Here's how the part is built. I have some questions about the finished solid (model axes, mm). Face numbers are marked on the shaded views. Give positions to 0.01 mm unless a question says otherwise; leave off trailing zeros. Write each loop counter-clockwise with the first axis right and the second up, starting at its lowest first coordinate (ties: lowest second). Pieces come first, ordered by that corner, then holes. Notation, with made-up numbers: (51, 27) - (97, 27) arc R33 ccw to (97, 60) - close; hole circle Ø3 at (77.5, -33.75). An arc over 180 degrees is marked (long way). Use a Markdown table: item, result.
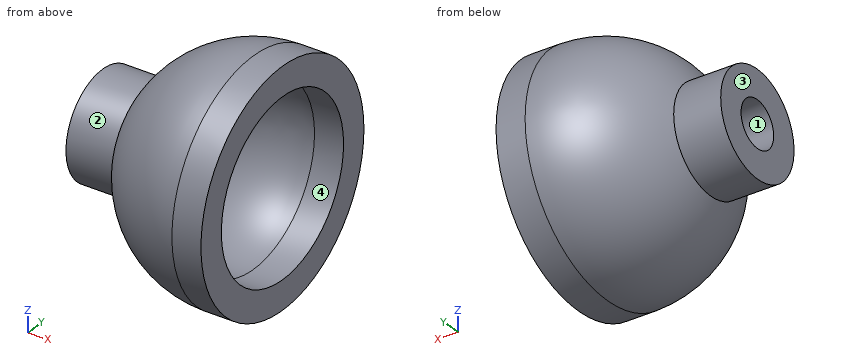
```python
from build123d import *


with BuildPart() as part:
    # Sketch1 → Revolve1 (revolve)
    with BuildSketch(Plane.XY):
        with BuildLine():
            Line((-10.380317683, 1.6), (-7.838367177, 1.6))
            Line((-7.838367177, 1.6), (-5.782732918, 1.6))
            ThreePointArc((-5.782732918, 1.6), (-3.633180425, 4.774934555), (0, 6))
            Line((0, 6), (2, 6))
            Line((2, 6), (2, 8))
            Line((2, 8), (0, 8))
            ThreePointArc((0, 8), (-4.195235393, 6.811754546), (-7.14422844, 3.6))
            Line((-7.14422844, 3.6), (-10.380317683, 3.6))
            Line((-10.380317683, 3.6), (-10.380317683, 1.6))
        make_face()
    revolve(axis=Axis((-14.839725853, 0, 0), (1, 0, 0)))


solid = part.part
```
Item 1: I need wall thicknesses on line 1 along Z through (x, y) = (-9.2, 0); line 2 along Z through (x, y) = (1.4, 0); line 3 along Y through (x, z) = (1, 5) (3 decimals). Which ranges of each line are inside material? Lowest first, please. Write a range as [from, to].
Values:
| item | result |
|---|---|
| line 1 | z = [-3.6, -1.6], [1.6, 3.6] |
| line 2 | z = [-8, -6], [6, 8] |
| line 3 | y = [-6.245, -3.317], [3.317, 6.245] |
Item 2: Thinking about a two-plate mould opening in Z: for the marked faces 1, 2, 3 and 4, which applies, +Z half, -Z half, draft (parallel to the pull), parting line (faces both ways), or undercut?
Values:
| item | result |
|---|---|
| face 1 | undercut |
| face 2 | parting line |
| face 3 | draft |
| face 4 | undercut |
Item 3: Will these pins go through, and if not, where does the flat tip stop? pin 1 Ø9.5 at (y, z) = (0, 0) entering from -X; pin 2 Ø3 at (x, z) = (-8.5, 0.5) entering from -Y; pin 3 Ø1.5 at (x, y) = (-3, 0.5) entering from -Z; pin 4 Ø3.5 at (y, z) = (0, 0) entering from +X.
Values:
| item | result |
|---|---|
| pin 1 | stops at x = -10.38 |
| pin 2 | stops at y = -3.85 |
| pin 3 | stops at z = -7.66 |
| pin 4 | stops at x = -5.74 |
Item 4: If we section it at D-D, the plane x = -9.25: Write out the boundary of the cut face in (y, z).
Values:
| item | result |
|---|---|
| outline | circle Ø7.2 at (0, 0); hole circle Ø3.2 at (0, 0) |
Item 5: If we section it at A-A, the plane y = 0: Write out the boundary of the cut face in (x, z), plus the area to 3 significant figures.
Values:
| item | result |
|---|---|
| outline | (-10.38, -3.6) - (-7.14, -3.6) arc R8 ccw to (0, -8) - (2, -8) - (2, -6) - (0, -6) arc R6 cw to (-5.78, -1.6) - (-10.38, -1.6) - close; (-10.38, 1.6) - (-5.78, 1.6) arc R6 cw to (0, 6) - (2, 6) - (2, 8) - (0, 8) arc R8 ccw to (-7.14, 3.6) - (-10.38, 3.6) - close |
| area | 56.9 mm2 |
Item 6: If we section it at C-C, the plane z = -2: Write out the boundary of the cut face in (x, y), plus the area to 3 significant figures.
Values:
| item | result |
|---|---|
| outline | (-10.38, -2.99) - (-7.14, -2.99) arc R7.75 ccw to (0, -7.75) - (2, -7.75) - (2, -5.66) - (0, -5.66) arc R5.66 cw to (0, 5.66) - (2, 5.66) - (2, 7.75) - (0, 7.75) arc R7.75 ccw to (-7.14, 2.99) - (-10.38, 2.99) - close |
| area | 69.3 mm2 |
